from build123d import *

# Parameters (mm, degrees)
SKETCH1_W                                 = 80
SKETCH1_H                                 = 60
BOSS_EXTRUDE1_DEPTH                       = 100
CUT_EXTRUDE1_START                        = 5
SKETCH2_W                                 = 35
SKETCH2_H                                 = 55
CUT_EXTRUDE1_DEPTH                        = 95
SKETCH3_W                                 = 80
SKETCH3_H                                 = 5
BOSS_EXTRUDE2_DEPTH                       = 70
BOSS_EXTRUDE3_DEPTH                       = 10
SKETCH5_W                                 = 20
SKETCH5_H                                 = 2.5
CUT_EXTRUDE2_DEPTH                        = 7.5
SKETCH6_W                                 = 35
SKETCH6_H                                 = 12
CUT_EXTRUDE4_DEPTH                        = 57.5
CUT_EXTRUDE6_REACH                        = 184.483
SKETCH7_R                                 = 4
SKETCH9_W                                 = 80
SKETCH9_H                                 = 50
BOSS_EXTRUDE4_DEPTH                       = 5
SKETCH13_W                                = 8
SKETCH13_H                                = 7
CUT_EXTRUDE8_BUTTON_HOLES_DEPTH           = 166.90660023
BOSS_EXTRUDE5_OLED_MOUNT_DEPTH            = 10
BOSS_EXTRUDE6_OLED_MOUNT_DEPTH            = 1
BOSS_EXTRUDE7_START                       = -2.5
BOSS_EXTRUDE7_OLED_MOUNT_DEPTH            = 1
BOSS_EXTRUDE8_OLED_MOUNT_DEPTH            = 1
BOSS_EXTRUDE13_OLED_MOUNT_SUPPORT_DEPTH   = 30
CUT_EXTRUDE9_OLED_CABLE_DEPTH             = 10
CUT_EXTRUDE9_OLED_CABLE_DEPTH_BACK        = 154.430766146
SKETCH18_W                                = 2.36
SKETCH18_H                                = 8
BOSS_EXTRUDE12_OLED_CABLE_GUIDE_REACH     = 162.39
SKETCH20_W                                = 10
SKETCH20_H                                = 10
CUT_EXTRUDE10_SOLENOID_WIRE_HOLE_DEPTH    = 166.90660023
SKETCH21_W                                = 5
SKETCH21_H                                = 32
BOSS_EXTRUDE9_SOLENOID_SIDE_SUPPORT_DEPTH = 13
CHAMFER3_THUMB_SIZE                       = 2.5
CHAMFER5_THUMB_SIZE                       = 4.5
CHAMFER5_THUMB_SIZE2                      = 7.794228634
CHAMFER5_THUMB_PART_2_SIZE                = 4.5
CHAMFER5_THUMB_PART_2_SIZE2               = 7.794228634
CHAMFER5_THUMB_PART_3_SIZE                = 4.5
CHAMFER5_THUMB_PART_3_SIZE2               = 7.794228634
BOSS_EXTRUDE5_GUIDE_DEPTH                 = 180
SKETCH49_W                                = 5
SKETCH49_H                                = 5
BOSS_EXTRUDE14_DEPTH                      = 5
CHAMFER8_SIZE                             = 5


with BuildPart() as part:
    # Sketch1 → Boss-Extrude1 (new body)
    with BuildSketch(Plane(origin=(0, 0, 0), x_dir=(1, 0, 0), z_dir=(0, 1, 0))):
        with Locations((40, 30)):
            Rectangle(SKETCH1_W, SKETCH1_H)
    extrude(amount=BOSS_EXTRUDE1_DEPTH)

    # Sketch2 → Cut-Extrude1 (cut)
    with BuildSketch(Plane(origin=(0, 0, 0), x_dir=(1, 0, 0), z_dir=(0, 1, 0)).offset(CUT_EXTRUDE1_START)):
        with Locations((20, 30)):
            Rectangle(SKETCH2_W, SKETCH2_H)
        with Locations((60, 30)):
            Rectangle(SKETCH2_W, SKETCH2_H)
    extrude(amount=CUT_EXTRUDE1_DEPTH, mode=Mode.SUBTRACT)

    # Sketch3 → Boss-Extrude2 (add)
    with BuildSketch(Plane.XY):
        with Locations((40, 2.5)):
            Rectangle(SKETCH3_W, SKETCH3_H)
    extrude(amount=BOSS_EXTRUDE2_DEPTH)

    # Sketch4 → Boss-Extrude3 (add)
    with BuildSketch(Plane(origin=(0, 5, 0), x_dir=(1, 0, 0), z_dir=(0, 1, 0))):
        Polygon((80, 0), (77.5, 0), (77.5, -67.5), (42.5, -67.5), (42.5, 0), (37.5, 0), (37.5, -67.5), (2.5, -67.5), (2.5, 0), (0, 0), (0, -70), (80, -70), align=None)
    extrude(amount=BOSS_EXTRUDE3_DEPTH)

    # Sketch5 → Cut-Extrude2 (cut)
    with BuildSketch(Plane(origin=(0, 15, 0), x_dir=(1, 0, 0), z_dir=(0, 1, 0))):
        with Locations((20, -68.75)):
            Rectangle(SKETCH5_W, SKETCH5_H)
        with Locations((60, -68.75)):
            Rectangle(SKETCH5_W, SKETCH5_H)
    extrude(amount=-CUT_EXTRUDE2_DEPTH, mode=Mode.SUBTRACT)

    # Sketch6 → Cut-Extrude4 (cut)
    with BuildSketch(Plane.XY):
        with Locations((20, 11)):
            Rectangle(SKETCH6_W, SKETCH6_H)
        with Locations((60, 11)):
            Rectangle(SKETCH6_W, SKETCH6_H)
    extrude(amount=-CUT_EXTRUDE4_DEPTH, mode=Mode.SUBTRACT)

    # Sketch7 → Cut-Extrude6 (cut, up to next)
    with BuildSketch(Plane(origin=(0, 0, -60), x_dir=(-1, 0, 0), z_dir=(0, 0, -1)), mode=Mode.PRIVATE) as cut_extrude6_sk1:
        with Locations((-20, 11.5)):
            Circle(SKETCH7_R)
    cut_extrude6_tool1 = extrude(cut_extrude6_sk1.sketch, amount=-CUT_EXTRUDE6_REACH, mode=Mode.PRIVATE) & part.part
    # Sketch7 → Cut-Extrude6 (cut, up to next)
    with BuildSketch(Plane(origin=(0, 0, -60), x_dir=(-1, 0, 0), z_dir=(0, 0, -1)), mode=Mode.PRIVATE) as cut_extrude6_sk2:
        with Locations((-60, 11.5)):
            Circle(SKETCH7_R)
    cut_extrude6_tool2 = extrude(cut_extrude6_sk2.sketch, amount=-CUT_EXTRUDE6_REACH, mode=Mode.PRIVATE) & part.part
    add(cut_extrude6_tool1.solids().sort_by_distance((20, 11.5, -60))[0], mode=Mode.SUBTRACT)
    add(cut_extrude6_tool2.solids().sort_by_distance((60, 11.5, -60))[0], mode=Mode.SUBTRACT)

    # Sketch9 → Boss-Extrude4 (add)
    with BuildSketch(Plane(origin=(0, 0, 0), x_dir=(1, 0, 0), z_dir=(0, 1, 0))):
        with Locations((40, 85)):
            Rectangle(SKETCH9_W, SKETCH9_H)
    extrude(amount=BOSS_EXTRUDE4_DEPTH)

    # Sketch13 → Cut-Extrude8 (Button Holes) (cut, through all)
    with BuildSketch(Plane(origin=(0, 5, 0), x_dir=(1, 0, 0), z_dir=(0, 1, 0))):
        with Locations((20, -61)):
            Rectangle(SKETCH13_W, SKETCH13_H)
        with Locations((60, -61)):
            Rectangle(SKETCH13_W, SKETCH13_H)
    extrude(amount=-CUT_EXTRUDE8_BUTTON_HOLES_DEPTH, mode=Mode.SUBTRACT)

    # Sketch14 → Boss-Extrude5 (OLED Mount) (add)
    with BuildSketch(Plane.XY):
        Polygon((25, 100), (26, 100), (26, 71), (54, 71), (54, 100), (55, 100), (55, 70), (54, 70), (26, 70), (25, 70), align=None)
    extrude(amount=BOSS_EXTRUDE5_OLED_MOUNT_DEPTH)

    # Sketch15 → Boss-Extrude6 (OLED Mount) (add)
    with BuildSketch(Plane.XY.offset(10)):
        Polygon((26, 71), (34, 71), (26, 75), align=None)
        Polygon((54, 75), (54, 71), (46, 71), align=None)
    extrude(amount=-BOSS_EXTRUDE6_OLED_MOUNT_DEPTH)

    # Sketch15<2> → Boss-Extrude7 (OLED Mount) (add)
    with BuildSketch(Plane.XY.offset(10).offset(BOSS_EXTRUDE7_START)):
        Polygon((26, 71), (34, 71), (26, 75), align=None)
        Polygon((54, 75), (54, 71), (46, 71), align=None)
    extrude(amount=-BOSS_EXTRUDE7_OLED_MOUNT_DEPTH)

    # Sketch17 → Boss-Extrude8 (OLED Mount) (add)
    with BuildSketch(Plane.XY.offset(10)):
        Polygon((54, 95), (54, 100), (46, 100), align=None)
        Polygon((26, 100), (34, 100), (26, 95), align=None)
    extrude(amount=-BOSS_EXTRUDE8_OLED_MOUNT_DEPTH)

    # Sketch32 → Boss-Extrude13 OLED Mount Support) (add)
    with BuildSketch(Plane.ZY.offset(-25)):
        Polygon((0, 70), (10, 70), (0, 60), align=None)
    extrude(amount=-BOSS_EXTRUDE13_OLED_MOUNT_SUPPORT_DEPTH)

    # Sketch18 → Cut-Extrude9 (OLED Cable) (cut, two sides: drawn at the far end of the back side and taken through both)
    with BuildSketch(Plane(origin=(0, 71, 0), x_dir=(1, 0, 0), z_dir=(0, 1, 0)).offset(-CUT_EXTRUDE9_OLED_CABLE_DEPTH_BACK)):
        with Locations((40, -1)):
            Rectangle(SKETCH18_W, SKETCH18_H)
    extrude(amount=CUT_EXTRUDE9_OLED_CABLE_DEPTH + CUT_EXTRUDE9_OLED_CABLE_DEPTH_BACK, mode=Mode.SUBTRACT)

    # Boss-Extrude12 (OLED Cable Guide): up to this plane
    boss_extrude12_oled_cable_guide_end = Plane(origin=(55, 70, 10), z_dir=(0, -0.7071067811865477, 0.7071067811865474))
    # Sketch31 → Boss-Extrude12 (OLED Cable Guide) (add, up to the surface)
    with BuildSketch(Plane(origin=(0, 15, 0), x_dir=(1, 0, 0), z_dir=(0, 1, 0)), mode=Mode.PRIVATE) as boss_extrude12_oled_cable_guide_sk1:
        Polygon((37.5, 0), (38.82, 0), (38.82, -5), (41.18, -5), (41.18, 0), (42.5, 0), (42.5, -7), (37.5, -7), align=None)
    boss_extrude12_oled_cable_guide_tool1 = split(extrude(boss_extrude12_oled_cable_guide_sk1.sketch, amount=BOSS_EXTRUDE12_OLED_CABLE_GUIDE_REACH, mode=Mode.PRIVATE), bisect_by=boss_extrude12_oled_cable_guide_end, keep=Keep.BOTH, mode=Mode.PRIVATE)
    add(boss_extrude12_oled_cable_guide_tool1.solids().sort_by_distance((38.16, 15, 0.086023))[0])

    # Sketch20 → Cut-Extrude10 (Solenoid Wire Hole) (cut, through all)
    with BuildSketch(Plane(origin=(0, 5, 0), x_dir=(1, 0, 0), z_dir=(0, 1, 0))):
        with Locations((60, 65)):
            Rectangle(SKETCH20_W, SKETCH20_H)
        with Locations((20, 65)):
            Rectangle(SKETCH20_W, SKETCH20_H)
    extrude(amount=-CUT_EXTRUDE10_SOLENOID_WIRE_HOLE_DEPTH, mode=Mode.SUBTRACT)

    # Sketch21 → Boss-Extrude9 (Solenoid Side Support) (add)
    with BuildSketch(Plane(origin=(0, 5, 0), x_dir=(1, 0, 0), z_dir=(0, 1, 0))):
        with Locations((70, 76)):
            Rectangle(SKETCH21_W, SKETCH21_H)
        with Locations((50, 76)):
            Rectangle(SKETCH21_W, SKETCH21_H)
        with Locations((30, 76)):
            Rectangle(SKETCH21_W, SKETCH21_H)
        with Locations((10, 76)):
            Rectangle(SKETCH21_W, SKETCH21_H)
    extrude(amount=BOSS_EXTRUDE9_SOLENOID_SIDE_SUPPORT_DEPTH)

    # Chamfer3 (Thumb)
    chamfer3_thumb_edges = [part.edges().sort_by_distance(p)[0] for p in [
        (20, 7.5, 67.5),
        (60, 7.5, 67.5),
    ]]
    chamfer(chamfer3_thumb_edges, length=CHAMFER3_THUMB_SIZE - 0.0001)  # a hair under: the kernel refuses the full size

    # Chamfer5 (Thumb)
    chamfer5_thumb_edges = [part.edges().sort_by_distance(p)[0] for p in [
        (70, 15, 68.75),
    ]]
    chamfer5_thumb_side = [part.faces().sort_by_distance(p)[0] for p in [
        (78.266129032, 15, 38.266129032),
    ]]
    chamfer(chamfer5_thumb_edges, length=CHAMFER5_THUMB_SIZE, length2=CHAMFER5_THUMB_SIZE2, reference=chamfer5_thumb_side[0])

    # Chamfer5 (Thumb) part 2
    chamfer5_thumb_part_2_edges = [part.edges().sort_by_distance(p)[0] for p in [
        (50, 15, 68.75),
        (30, 15, 68.75),
    ]]
    chamfer5_thumb_part_2_side = [part.faces().sort_by_distance(p)[0] for p in [
        (40, 15, 41.718085106),
    ]]
    chamfer(chamfer5_thumb_part_2_edges, length=CHAMFER5_THUMB_PART_2_SIZE, length2=CHAMFER5_THUMB_PART_2_SIZE2, reference=chamfer5_thumb_part_2_side[0])

    # Chamfer5 (Thumb) part 3
    chamfer5_thumb_part_3_edges = [part.edges().sort_by_distance(p)[0] for p in [
        (10, 15, 68.75),
    ]]
    chamfer5_thumb_part_3_side = [part.faces().sort_by_distance(p)[0] for p in [
        (1.733870968, 15, 38.266129032),
    ]]
    chamfer(chamfer5_thumb_part_3_edges, length=CHAMFER5_THUMB_PART_3_SIZE, length2=CHAMFER5_THUMB_PART_3_SIZE2, reference=chamfer5_thumb_part_3_side[0])

    # Sketch37 → Boss-Extrude5 (Guide) (add, through all)
    with BuildSketch(Plane.XY.offset(70)):
        Polygon((80, 0), (83, 0), (80, 3), align=None)
        Polygon((0, 0), (-3, 0), (0, 3), align=None)
    extrude(amount=-BOSS_EXTRUDE5_GUIDE_DEPTH)

    # Sketch49 → Boss-Extrude14 (add)
    with BuildSketch(Plane(origin=(0, 15, 0), x_dir=(1, 0, 0), z_dir=(0, 1, 0))):
        with Locations((40, -9.5)):
            Rectangle(SKETCH49_W, SKETCH49_H)
    extrude(amount=BOSS_EXTRUDE14_DEPTH)

    # Chamfer8
    chamfer8_edges = [part.edges().sort_by_distance(p)[0] for p in [
        (40, 20, 12),
    ]]
    chamfer(chamfer8_edges, length=CHAMFER8_SIZE - 0.0001)  # a hair under: the kernel refuses the full size


solid = part.part
Verification items for the finished model (mm, model axes). A direction names the side the tool comes from. Give positions to 0.01 mm unless a question says otherwise; leave off trailing zeros. Loops run counter-clockwise (first coordinate to the right, second up) from the corner with the lowest first, then second, coordinate; pieces in that order, holes last.
1. Cross-section at D-D on y = 37. Record the cut outline in (x, z).
Derived:
outline: (0, -60) - (80, -60) - (80, 0) - (42.5, 0) - (42.5, 7) - (37.5, 7) - (37.5, 0) - (0, 0) - close; hole (2.5, -57.5) - (37.5, -57.5) - (37.5, -2.5) - (2.5, -2.5) - close; hole (38.82, -3) - (41.18, -3) - (41.18, 5) - (38.82, 5) - close; hole (42.5, -57.5) - (77.5, -57.5) - (77.5, -2.5) - (42.5, -2.5) - close
2. Material ranges on probe 1 along X at (y, z) = (11, -59); probe 2 along X at (y, z) = (42, -12); probe 3 along Z at (x, y) = (56, 47), recorded low to high.
Derived:
probe 1: x = 0 to 16.03, 23.97 to 56.03, 63.97 to 80
probe 2: x = 0 to 2.5, 37.5 to 42.5, 77.5 to 80
probe 3: z = -60 to -57.5, -2.5 to 0
3. Cross-section at C-C on y = 89. Record the cut outline in (x, z), and give its area (3 significant figures).
Derived:
outline: (0, -60) - (80, -60) - (80, 0) - (55, 0) - (55, 10) - (54, 10) - (54, 0) - (26, 0) - (26, 10) - (25, 10) - (25, 0) - (0, 0) - close; hole (2.5, -57.5) - (37.5, -57.5) - (37.5, -2.5) - (2.5, -2.5) - close; hole (42.5, -57.5) - (77.5, -57.5) - (77.5, -2.5) - (42.5, -2.5) - close
area: 970 mm2
4. Release check for a two-part mould opening along Z. For faces 1 (the flat face through (30.056, 97.535, 9.507)), 2 (the flat face through (30.5, 7.4, 67.5)), 3 (the flat face through (70, 11, -92)), 4 (the flat face through (65, 57, 0)) record: +Z half, -Z half, draft (parallel to the pull), parting line (faces both ways), or undercut.
Derived:
face 1: draft
face 2: undercut
face 3: -Z half
face 4: +Z half
5. Tool access check on faces 5 (the flat face through (80, 40, -39)), 6 (the flat face through (60, 3, 64.5)), 7 (the flat face through (40, 18, 9)), 8 (the flat face through (30, 18, -76)). Record the directions out of +Z, -Z, +X, -X, +Y, -Y that give a thin tool (end or side, any length) a straight path to the whole face; none if there is none.
Derived:
face 5: +Z, -Z, +X, +Y
face 6: +Y, -Y
face 7: +Z, +X, -X
face 8: -Z, +X, -X, +Y
6. Cross-section at B-B on z = -82.5. Record the cut outline in (x, y).
Derived:
outline: (-3, 0) - (83, 0) - (80, 3) - (80, 5) - (72.5, 5) - (72.5, 18) - (67.5, 18) - (67.5, 5) - (52.5, 5) - (52.5, 18) - (47.5, 18) - (47.5, 5) - (32.5, 5) - (32.5, 18) - (27.5, 18) - (27.5, 5) - (12.5, 5) - (12.5, 18) - (7.5, 18) - (7.5, 5) - (0, 5) - (0, 3) - close
7. Go/stop test with flat-tipped pins: P1, Ø4, axis at x = 7, y = 77.5, coming from the -Z side; P2, Ø2.5, axis at y = 56, z = -0.5, coming from the -X side; P3, Ø2, axis at x = 51.5, y = 73.5, coming from the +Z side. Record where each tip stops, or that it passes through.
Derived:
P1: stops at z = -60
P2: stops at x = 0
P3: stops at z = 10
8. Cross-section at A-A on x = 20. Count the separate pieces of the cut face and the enclosed holes in it, and give its area (3 significant figures).
Derived:
separate pieces: 5
enclosed holes: 0
area: 1,240 mm2
